Job drawing, mm, ordinate dimensions from the low corner. One solid piece. A direction names the side the tool comes from. Coordinates: 2 decimals unless noted, no trailing zeros. Order: outer loops, then holes, each group sorted by start corner. A loop starts at its lowest first (then second) coordinate and runs counter-clockwise, first axis right, second up. Notation, with made-up numbers: (80, -36.5) - (136, -36.5) arc R18 ccw to (136, -6.5) - close; hole circle Ø9 at (22, 25.5). An arc over 180 degrees is marked (long way). Return JSON: item names as keys, results as strings.
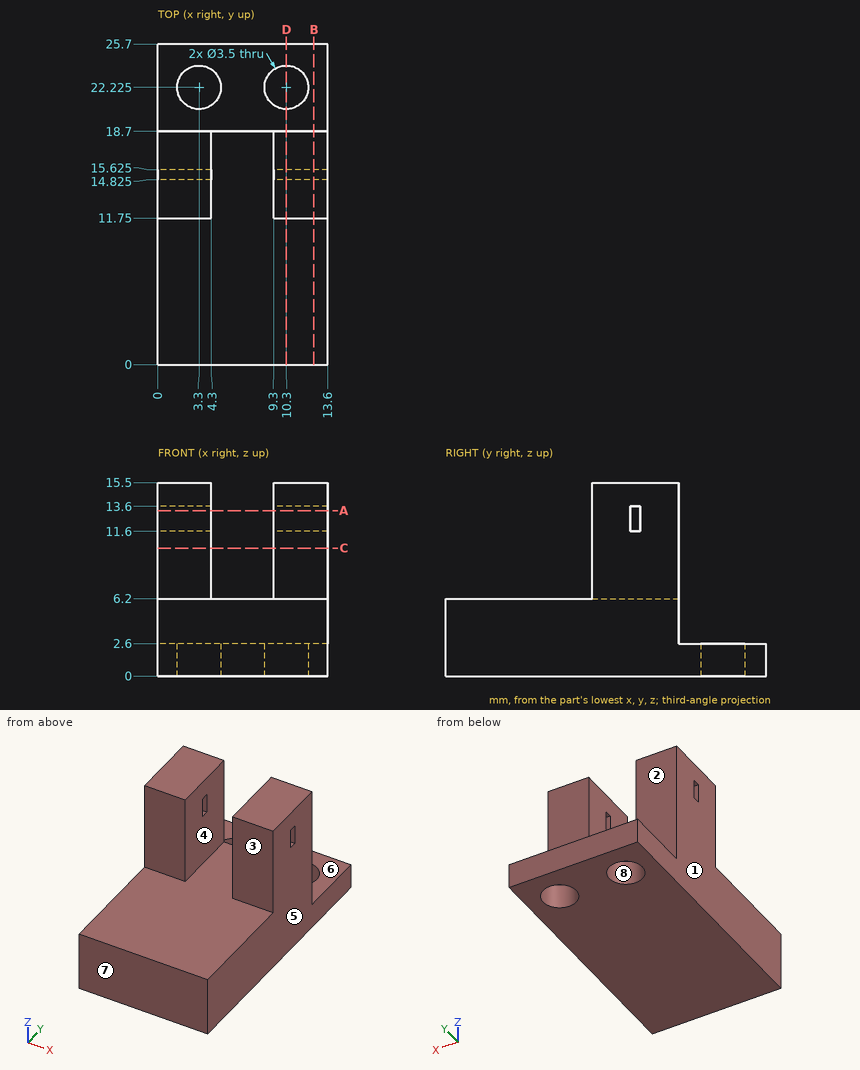
1. Cut at D-D on x = 10.3. Give the cut face in (y, z) (3 decimals), plus the area to 3 significant figures.
Check values:
{"outline": "(0, 0) - (20.475, 0) - (20.475, 2.6) - (18.7, 2.6) - (18.7, 15.5) - (11.75, 15.5) - (11.75, 6.2) - (0, 6.2) - close; (23.975, 0) - (25.7, 0) - (25.7, 2.6) - (23.975, 2.6) - close; hole (14.825, 11.6) - (15.625, 11.6) - (15.625, 13.6) - (14.825, 13.6) - close", "area": "188 mm²"}
2. Probe L1, parallel to Y at x = 3.3, z = 1.9 (3 decimals); L2, parallel to X at y = 13.25, z = 8; L3, parallel to Y at x = 4, z = 12.25 (3 decimals). List the from-to ranges inside material, lowest first.
Check values:
{"L1": "0 to 20.475, 23.975 to 25.7", "L2": "0 to 4.3, 9.3 to 13.6", "L3": "11.75 to 14.825, 15.625 to 18.7"}
3. Cut at C-C on z = 10.25. Give the cut face in (x, y), plus the area to 3 significant figures.
Check values:
{"outline": "(0, 11.75) - (4.3, 11.75) - (4.3, 18.7) - (0, 18.7) - close; (9.3, 11.75) - (13.6, 11.75) - (13.6, 18.7) - (9.3, 18.7) - close", "area": "59.8 mm²"}
4. Tool access for the marked faces 1, 2, 3, 4 and 5: list every direction of +Z, -Z, +X, -X, +Y, -Y with a clear straight run to the whole face (end or side of a thin tool).
Check values:
{"face 1": "+Z, -Z, -X, +Y, -Y", "face 2": "+Z, +X, -X, +Y", "face 3": "+Z, +X, -X, -Y", "face 4": "+Z, +Y, -Y", "face 5": "+Z, -Z, +X, +Y, -Y"}
5. Drop flat-ended pins along their axis: pin 1 (4.5 mm diameter, centred on x = 11.5, z = 9, fed in from -Y); pin 2 (5.5 mm diameter, centred on x = 7, y = 22, fed in from +Z); pin 3 (1 mm diameter, centred on x = 1.5, z = 12, fed in from +Y). Give the stop position or say it passes through.
Check values:
{"pin 1": "y = 11.75", "pin 2": "z = 2.6", "pin 3": "y = 18.7"}
6. Cut at A-A on z = 13.25. Give the cut face in (x, y) (3 decimals).
Check values:
{"outline": "(0, 11.75) - (4.3, 11.75) - (4.3, 14.825) - (0, 14.825) - close; (0, 15.625) - (4.3, 15.625) - (4.3, 18.7) - (0, 18.7) - close; (9.3, 11.75) - (13.6, 11.75) - (13.6, 14.825) - (9.3, 14.825) - close; (9.3, 15.625) - (13.6, 15.625) - (13.6, 18.7) - (9.3, 18.7) - close"}
7. Mould opens along Y. For the marked faces 6, 7 and 8 say: pulls with the +Y half, pulls with the -Y half, needs draft (parallel to the pull), parting line crosses it, or undercut.
Check values:
{"face 6": "needs draft", "face 7": "pulls with the -Y half", "face 8": "undercut"}
8. Cut at B-B on x = 12.5. Give the cut face in (y, z) (3 decimals), plus the area to 3 significant figures.
Check values:
{"outline": "(0, 0) - (25.7, 0) - (25.7, 2.6) - (18.7, 2.6) - (18.7, 15.5) - (11.75, 15.5) - (11.75, 6.2) - (0, 6.2) - close; hole (14.825, 11.6) - (15.625, 11.6) - (15.625, 13.6) - (14.825, 13.6) - close", "area": "197 mm²"}
